from build123d import *

# Parameters (mm, degrees)
SKETCH_3_R          = 0.5
CUT_EXTRUDE_1_DEPTH = 10


with BuildPart() as part:
    # 草图2 → 旋转1 (revolve)
    with BuildSketch(Plane(origin=(0, 0, 0), x_dir=(0, 0, -1), z_dir=(1, 0, 0)), mode=Mode.PRIVATE) as revolve_1_sk:
        Polygon((0, 3.2), (3, 3.2), (3, 2.4), (4, 2.4), (4, 4), (0, 4), align=None)
    revolve(revolve_1_sk.sketch.rotate(Axis((0, 0, 0), (0, 0, -1)), 90), axis=Axis((0, 0, 0), (0, 0, -1)))

    # 草图3 → 切除-拉伸1 (cut)
    with BuildSketch(Plane(origin=(0, 0, 0), x_dir=(1, 0, 0), z_dir=(0, 1, 0))):
        with Locations(Location((0, 1, 0), (0, 0, 270))):
            Circle(SKETCH_3_R)
    extrude(amount=-CUT_EXTRUDE_1_DEPTH, mode=Mode.SUBTRACT)


solid = part.part
Geometry check sheet. Reference: the model listing, model coordinates, mm. A direction names the side the tool comes from. Round coordinates to 2 decimals unless told otherwise and drop trailing zeros. Order: outer loops, then holes, each group sorted by start corner. A loop starts at its lowest first (then second) coordinate and runs counter-clockwise, first axis right, second up. Notation, with made-up numbers: M 50,45.25 L 63,45.25 A36 ccw 63,84.25 Z; hole C 35.5,-11.75 d6. An arc over 180 degrees is marked long. Answer in a Markdown table with one row per item.
(1) Sectioned sample at A-A, the plane y = 0. Record the cut outline in (x, z), and give its area (3 significant figures).
Responses:
| item | result |
|---|---|
| outline | M -4,-4 L -2.4,-4 L -2.4,-3 L -3.2,-3 L -3.2,0 L -4,0 Z; M 2.4,-4 L 4,-4 L 4,0 L 3.2,0 L 3.2,-3 L 2.4,-3 Z |
| area | 8.00 mm² |
(2) Sectioned sample at D-D, the plane z = -3.1. Record the cut outline in (x, y), and give its area (3 significant figures).
Responses:
| item | result |
|---|---|
| outline | C 0,0 d8; hole C 0,0 d4.8 |
| area | 32.2 mm² |
(3) Go/stop test with flat-tipped pins: P1, Ø2, axis at x = 1.5, z = -1, coming from the +Y side; P2, Ø1, axis at y = -1.5, z = -1.5, coming from the -X side. Record where each tip stops, or that it passes through.
Responses:
| item | result |
|---|---|
| P1 | stops at y = 3.97 |
| P2 | stops at x = -3.87 |
(4) Draft check along X on faces 3 (the face through (-0.3, -3.6, -1.4)), 4 (the face through (-2, 2, -4)), 5 (the face through (-0.867, 3.905, -1.972)). Enter one of: released by +X, released by -X, zero draft, split by the parting line, or undercut.
Responses:
| item | result |
|---|---|
| face 3 | undercut |
| face 4 | zero draft |
| face 5 | split by the parting line |
(5) Scan lines: probe 1 along Z at (x, y) = (0, -3.6); probe 2 along Z at (x, y) = (1, -2.75); probe 3 along Y at (x, z) = (-1, -0.7). Record each from-to range of solid material in increasing order. Write a range as from..to.
Responses:
| item | result |
|---|---|
| probe 1 | z = -4..-1.5, -0.5..0 |
| probe 2 | z = -4..-3 |
| probe 3 | y = -3.87..-3.04, 3.04..3.87 |
(6) Sectioned sample at B-B, the plane x = 0. Record the cut outline in (y, z).
Responses:
| item | result |
|---|---|
| outline | M -4,-4 L -2.4,-4 L -2.4,-3 L -3.2,-3 L -3.2,-1.5 L -4,-1.5 Z; M -4,-0.5 L -3.2,-0.5 L -3.2,0 L -4,0 Z; M 2.4,-4 L 4,-4 L 4,0 L 3.2,0 L 3.2,-3 L 2.4,-3 Z |
(7) Tool access check on faces 1 (the face through (-2, -3, 0)), 2 (the face through (1.477, 2.839, -1.521)). Record the directions out of +Z, -Z, +X, -X, +Y, -Y that give a thin tool (end or side, any length) a straight path to the whole face; none if there is none.
Responses:
| item | result |
|---|---|
| face 1 | +Z, +X, -X, +Y, -Y |
| face 2 | +Z |
(8) Sectioned sample at C-C, the plane x = -2.25. Record the cut outline in (y, z).
Responses:
| item | result |
|---|---|
| outline | M -3.31,-4 L -0.84,-4 L -0.84,-3 L -2.28,-3 L -2.28,0 L -3.31,0 Z; M 0.84,-4 L 3.31,-4 L 3.31,0 L 2.28,0 L 2.28,-3 L 0.84,-3 Z |
